Check sheet for the modelled part. Datum: model origin and axes. Units: mm. A direction names the side the tool comes from. Give positions to 0.01 mm unless a question says otherwise; leave off trailing zeros. Loops run counter-clockwise (first coordinate to the right, second up) from the corner with the lowest first, then second, coordinate; pieces in that order, holes last. Notation, with made-up numbers: M -30,-34 L 3,-34 A8 cw 3,-26 Z; hole C 84.5,41 d1. An arc over 180 degrees is marked long. Use one line per item in the form item = value.
from build123d import *

# Parameters (mm, degrees)
SKETCH2_R               = 50.8
SKETCH2_R_2             = 41.275
BASE_CYLINDER_DEPTH     = 292.1
SKETCH3_R               = 69.85
SKETCH3_R_2             = 41.275
AFT_FLANGE_DEPTH        = 17.78
SKETCH4_R               = 69.85
SKETCH4_R_2             = 41.275
FORWARD_FLANGE_DEPTH    = 17.78
SKETCH6_R               = 50.0761
SKETCH6_R_2             = 47.0027
O_RING_SLOT_1_DEPTH     = 1.9812
SKETCH7_R               = 50.0761
SKETCH7_R_2             = 47.0027
O_RING_SLOT_2_DEPTH     = 1.9812
SKETCH8_R               = 3.175
CUT_EXTRUDE4_DEPTH      = 1
CUT_EXTRUDE4_DEPTH_BACK = 293.1
FILLET1_R               = 4.7625
SKETCH9_R               = 3.175
CUT_EXTRUDE5_DEPTH      = 7.62
SKETCH10_R              = 3.175
CUT_EXTRUDE6_DEPTH      = 7.62
CUT_EXTRUDE7_REACH      = 286.48
SKETCH11_R              = 1.4097
CUT_EXTRUDE8_REACH      = 286.48
SKETCH12_R              = 1.4097
SKETCH13_R              = 2.3114
CUT_EXTRUDE10_DEPTH     = 6.35
SKETCH14_R              = 2.3114
CUT_EXTRUDE11_DEPTH     = 6.35


with BuildPart() as part:
    # Sketch2 → Base Cylinder (new body)
    with BuildSketch(Plane(origin=(0, 0, 0), x_dir=(1, 0, 0), z_dir=(0, 1, 0))):
        Circle(SKETCH2_R)
        Circle(SKETCH2_R_2, mode=Mode.SUBTRACT)
    extrude(amount=BASE_CYLINDER_DEPTH)

    # Sketch3 → Aft Flange (add)
    with BuildSketch(Plane.XZ):
        Circle(SKETCH3_R)
        Circle(SKETCH3_R_2, mode=Mode.SUBTRACT)
    extrude(amount=-AFT_FLANGE_DEPTH)

    # Sketch4 → Forward Flange (add)
    with BuildSketch(Plane(origin=(0, 292.1, 0), x_dir=(1, 0, 0), z_dir=(0, 1, 0))):
        Circle(SKETCH4_R)
        Circle(SKETCH4_R_2, mode=Mode.SUBTRACT)
    extrude(amount=-FORWARD_FLANGE_DEPTH)

    # Sketch6 → O-Ring Slot 1 (cut)
    with BuildSketch(Plane.XZ):
        Circle(SKETCH6_R)
        Circle(SKETCH6_R_2, mode=Mode.SUBTRACT)
    extrude(amount=-O_RING_SLOT_1_DEPTH, mode=Mode.SUBTRACT)

    # Sketch7 → O-Ring Slot 2 (cut)
    with BuildSketch(Plane(origin=(0, 292.1, 0), x_dir=(1, 0, 0), z_dir=(0, 1, 0))):
        Circle(SKETCH7_R)
        Circle(SKETCH7_R_2, mode=Mode.SUBTRACT)
    extrude(amount=-O_RING_SLOT_2_DEPTH, mode=Mode.SUBTRACT)

    # Sketch8 → Cut-Extrude4 (cut, two sides)
    with BuildSketch(Plane.XZ) as cut_extrude4_sk:
        with Locations((-59.9186, 0)):
            Circle(SKETCH8_R)
        with Locations((-42.368848379, 42.368848379)):
            Circle(SKETCH8_R)
        with Locations((0, 59.9186)):
            Circle(SKETCH8_R)
        with Locations((42.368848379, 42.368848379)):
            Circle(SKETCH8_R)
        with Locations((59.9186, 0)):
            Circle(SKETCH8_R)
        with Locations((42.368848379, -42.368848379)):
            Circle(SKETCH8_R)
        with Locations((0, -59.9186)):
            Circle(SKETCH8_R)
        with Locations((-42.368848379, -42.368848379)):
            Circle(SKETCH8_R)
    extrude(amount=CUT_EXTRUDE4_DEPTH, mode=Mode.SUBTRACT)
    extrude(cut_extrude4_sk.sketch, amount=-CUT_EXTRUDE4_DEPTH_BACK, mode=Mode.SUBTRACT)

    # Fillet1
    fillet1_edges = [part.edges().sort_by_distance(p)[0] for p in [
        (-50.8, 17.78, 0),
        (-50.8, 274.32, 0),
    ]]
    fillet(fillet1_edges, radius=FILLET1_R)

    # Sketch9 → Cut-Extrude5 (cut)
    with BuildSketch(Plane(origin=(0, 292.1, 0), x_dir=(1, 0, 0), z_dir=(0, 1, 0))):
        with Locations((-22.929855511, 55.357568157)):
            Circle(SKETCH9_R)
        with Locations((22.929855511, -55.357568157)):
            Circle(SKETCH9_R)
        with Locations((22.929855511, 55.357568157)):
            Circle(SKETCH9_R)
        with Locations((-22.929855511, -55.357568157)):
            Circle(SKETCH9_R)
    extrude(amount=-CUT_EXTRUDE5_DEPTH, mode=Mode.SUBTRACT)

    # Sketch10 → Cut-Extrude6 (cut)
    with BuildSketch(Plane.XZ):
        with Locations((-22.929855511, 55.357568157)):
            Circle(SKETCH10_R)
        with Locations((22.929855511, -55.357568157)):
            Circle(SKETCH10_R)
        with Locations((22.929855511, 55.357568157)):
            Circle(SKETCH10_R)
        with Locations((-22.929855511, -55.357568157)):
            Circle(SKETCH10_R)
    extrude(amount=-CUT_EXTRUDE6_DEPTH, mode=Mode.SUBTRACT)

    # Sketch11 → Cut-Extrude7 (cut, up to next)
    with BuildSketch(Plane(origin=(0, 284.48, 0), x_dir=(1, 0, 0), z_dir=(0, 1, 0)), mode=Mode.PRIVATE) as cut_extrude7_sk1:
        with Locations((-22.929855511, 55.357568157)):
            Circle(SKETCH11_R)
    cut_extrude7_tool1 = extrude(cut_extrude7_sk1.sketch, amount=-CUT_EXTRUDE7_REACH, mode=Mode.PRIVATE) & part.part
    add(cut_extrude7_tool1.solids().sort_by_distance((-22.929856, 284.48, -55.357568))[0], mode=Mode.SUBTRACT)
    # Sketch11 → Cut-Extrude7 (cut, up to next)
    with BuildSketch(Plane(origin=(0, 284.48, 0), x_dir=(1, 0, 0), z_dir=(0, 1, 0)), mode=Mode.PRIVATE) as cut_extrude7_sk2:
        with Locations((22.929855511, 55.357568157)):
            Circle(SKETCH11_R)
    cut_extrude7_tool2 = extrude(cut_extrude7_sk2.sketch, amount=-CUT_EXTRUDE7_REACH, mode=Mode.PRIVATE) & part.part
    add(cut_extrude7_tool2.solids().sort_by_distance((22.929856, 284.48, -55.357568))[0], mode=Mode.SUBTRACT)
    # Sketch11 → Cut-Extrude7 (cut, up to next)
    with BuildSketch(Plane(origin=(0, 284.48, 0), x_dir=(1, 0, 0), z_dir=(0, 1, 0)), mode=Mode.PRIVATE) as cut_extrude7_sk3:
        with Locations((-22.929855511, -55.357568157)):
            Circle(SKETCH11_R)
    cut_extrude7_tool3 = extrude(cut_extrude7_sk3.sketch, amount=-CUT_EXTRUDE7_REACH, mode=Mode.PRIVATE) & part.part
    add(cut_extrude7_tool3.solids().sort_by_distance((-22.929856, 284.48, 55.357568))[0], mode=Mode.SUBTRACT)
    # Sketch11 → Cut-Extrude7 (cut, up to next)
    with BuildSketch(Plane(origin=(0, 284.48, 0), x_dir=(1, 0, 0), z_dir=(0, 1, 0)), mode=Mode.PRIVATE) as cut_extrude7_sk4:
        with Locations((22.929855511, -55.357568157)):
            Circle(SKETCH11_R)
    cut_extrude7_tool4 = extrude(cut_extrude7_sk4.sketch, amount=-CUT_EXTRUDE7_REACH, mode=Mode.PRIVATE) & part.part
    add(cut_extrude7_tool4.solids().sort_by_distance((22.929856, 284.48, 55.357568))[0], mode=Mode.SUBTRACT)

    # Sketch12 → Cut-Extrude8 (cut, up to next)
    with BuildSketch(Plane.XZ.offset(-7.62), mode=Mode.PRIVATE) as cut_extrude8_sk1:
        with Locations((-22.929855511, 55.357568157)):
            Circle(SKETCH12_R)
    cut_extrude8_tool1 = extrude(cut_extrude8_sk1.sketch, amount=-CUT_EXTRUDE8_REACH, mode=Mode.PRIVATE) & part.part
    add(cut_extrude8_tool1.solids().sort_by_distance((-22.929856, 7.62, 55.357568))[0], mode=Mode.SUBTRACT)
    # Sketch12 → Cut-Extrude8 (cut, up to next)
    with BuildSketch(Plane.XZ.offset(-7.62), mode=Mode.PRIVATE) as cut_extrude8_sk2:
        with Locations((22.929855511, 55.357568157)):
            Circle(SKETCH12_R)
    cut_extrude8_tool2 = extrude(cut_extrude8_sk2.sketch, amount=-CUT_EXTRUDE8_REACH, mode=Mode.PRIVATE) & part.part
    add(cut_extrude8_tool2.solids().sort_by_distance((22.929856, 7.62, 55.357568))[0], mode=Mode.SUBTRACT)
    # Sketch12 → Cut-Extrude8 (cut, up to next)
    with BuildSketch(Plane.XZ.offset(-7.62), mode=Mode.PRIVATE) as cut_extrude8_sk3:
        with Locations((-22.929855511, -55.357568157)):
            Circle(SKETCH12_R)
    cut_extrude8_tool3 = extrude(cut_extrude8_sk3.sketch, amount=-CUT_EXTRUDE8_REACH, mode=Mode.PRIVATE) & part.part
    add(cut_extrude8_tool3.solids().sort_by_distance((-22.929856, 7.62, -55.357568))[0], mode=Mode.SUBTRACT)
    # Sketch12 → Cut-Extrude8 (cut, up to next)
    with BuildSketch(Plane.XZ.offset(-7.62), mode=Mode.PRIVATE) as cut_extrude8_sk4:
        with Locations((22.929855511, -55.357568157)):
            Circle(SKETCH12_R)
    cut_extrude8_tool4 = extrude(cut_extrude8_sk4.sketch, amount=-CUT_EXTRUDE8_REACH, mode=Mode.PRIVATE) & part.part
    add(cut_extrude8_tool4.solids().sort_by_distance((22.929856, 7.62, -55.357568))[0], mode=Mode.SUBTRACT)

    # Sketch13 → Cut-Extrude10 (cut)
    with BuildSketch(Plane(origin=(-69.85, 0, 0), x_dir=(0, 0, -1), z_dir=(1, 0, 0))):
        with Locations((0, 283.21)):
            Circle(SKETCH13_R)
    extrude(amount=CUT_EXTRUDE10_DEPTH, mode=Mode.SUBTRACT)

    # Sketch14 → Cut-Extrude11 (cut)
    with BuildSketch(Plane(origin=(69.85, 0, 0), x_dir=(0, 0, -1), z_dir=(1, 0, 0))):
        with Locations((0, 283.21)):
            Circle(SKETCH14_R)
    extrude(amount=-CUT_EXTRUDE11_DEPTH, mode=Mode.SUBTRACT)


solid = part.part
1) Scan lines: line 1 (Z direction, x = -1.5, y = 270); line 2 (Y direction, x = -53, z = 32.5); line 3 (Y direction, x = 28, z = -39.5). Record each from-to range of solid material in increasing order.
Evaluation:
line_1 = -50.8 to -41.25, 41.25 to 50.8
line_2 = 0 to 17.78, 274.32 to 292.1
line_3 = 1.98 to 290.12
2) Section check B-B (y = 200.5). Record the cut outline in (x, z) (3 decimals).
Evaluation:
outline = C 0,0 d101.6; hole C 0,0 d82.55
3) Release check for a two-part mould opening along Z. For faces 4 (the face through (-55.431, 8.766, -42.503)), 5 (the face through (-22, 284.48, 57)), 6 (the face through (-52, 274.32, -21)) record: pulls with the +Z half, pulls with the -Z half, needs draft (parallel to the pull), parting line crosses it, or undercut.
Evaluation:
face_4 = parting line crosses it
face_5 = undercut
face_6 = needs draft
4) Set-up check for faces 1 (the face through (0, 292.1, 42)), 2 (the face through (-45, 290.119, 15)), 3 (the face through (25.863, 3.757, -56.574)): record each of +Z, -Z, +X, -X, +Y, -Y from which the full face is reachable in a straight line by a thin tool's end or side.
Evaluation:
face_1 = +Z, -Z, +X, -X, +Y
face_2 = +Y
face_3 = -Y
5) Depth check by flat-ended pin: pin 1 Ø1.5 at (x, y) = (37, 236) entering from +Z; pin 2 Ø2.5 at (y, z) = (283, 0.5) entering from -X; pin 3 Ø3 at (x, z) = (-23.5, 56.5) entering from +Y. Enter the tip coordinate at first touch or a pass-through.
Evaluation:
pin_1 = 35.59
pin_2 = -63.5
pin_3 = 284.48
6) Section check A-A (x = 0). State how many separate pieces and enclosed holes the cut face has, then the cut area to 3 significant figures.
Evaluation:
separate_pieces = 6
enclosed_holes = 0
area = 6,460 mm^2
